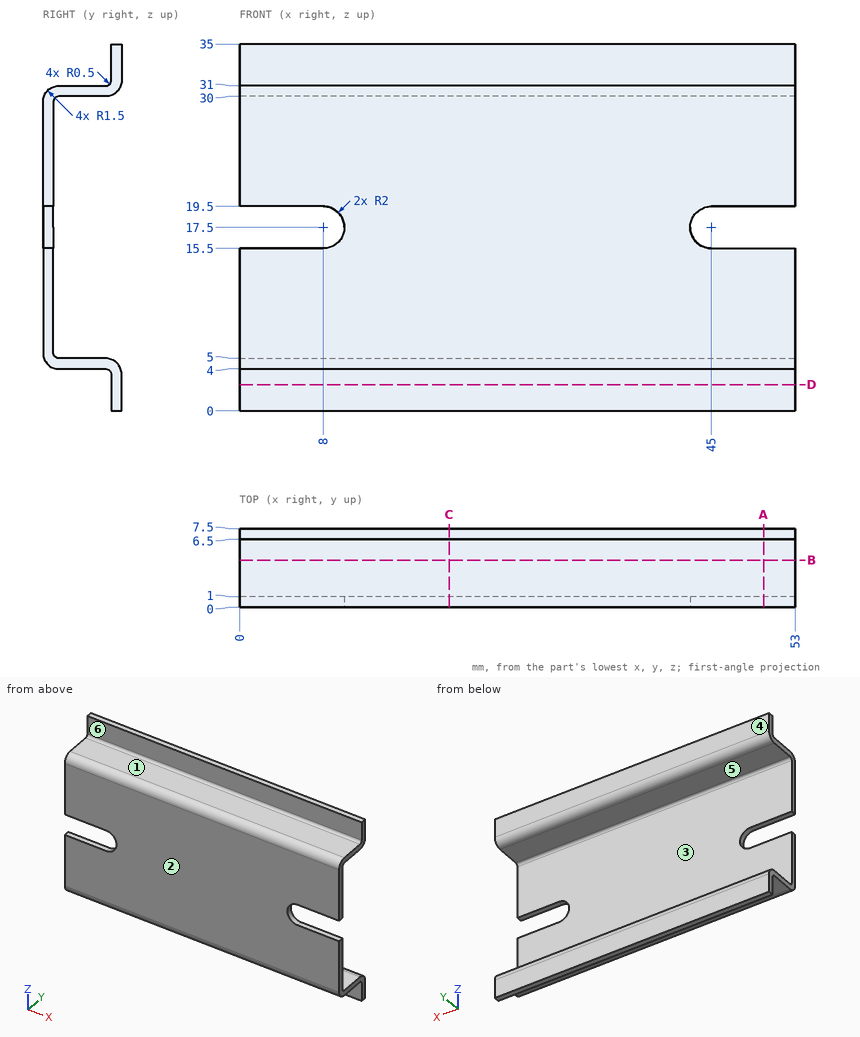
Study the drawing (mm; zero at the part's minimum x, y, z) and answer. A direction names the side the tool comes from. Coordinates: 2 decimals unless noted, no trailing zeros. Loops run counter-clockwise (first coordinate to the right, second up) from the corner with the lowest first, then second, coordinate; pieces in that order, holes last. Notation, with made-up numbers: M 23,20 L 34,20 A14 cw 34,41 Z; hole C 6.25,85 d8. An arc over 180 degrees is marked long. Answer in a Markdown table with one row per item. Add a question column.
1. Find section D-D, the plane z = 2.5. Write down the section's boundary in (x, y), then the cut area to 3 significant figures.
2. A tool of negligible diameter and unlimited length cuts with its end or side. For the marked faces 4, 5 and 6, from which of +Z, -Z, +X, -X, +Y, -Y can it reach the whole face along a straight path? Write none if from no direction.
3. Find section B-B, the plane y = 4.5. Write down the section's boundary in (x, z), then the cut area to 3 significant figures.
4. Consider L1, parallel to Z at x = 49, y = 4.25; L2, parallel to Y at x = 20, z = 26.5; L3, parallel to Z at x = 32, y = 1.25. Determine where each line is inside the solid, lowest interval first.
5. Find section C-C, the plane x = 20. Write down the section's boundary in (y, z).
6. Find section A-A, the plane x = 50. Write down the section's boundary in (y, z), then the cut area to 3 significant figures.
7. Flat-ended cylindrical pins translate along their axes: P1, Ø3.5, axis at x = 19.5, y = 3.5, coming from the +Z side; P2, Ø1, axis at x = 32.5, z = 2.5, coming from the -Y side; P3, Ø1.3, axis at x = 31, y = 3.5, coming from the -Z side. Find the tip coordinate at first contact, or state that the pin passes through.
8. The mould has two halves that part along Z. Classify the marked faces 1, 2 and 3: pulls with the +Z half, pulls with the -Z half, needs draft (parallel to the pull), parting line crosses it, or undercut.
Reported:
| question | item | result |
|---|---|---|
| 1 | outline | M 0,6.5 L 53,6.5 L 53,7.5 L 0,7.5 Z |
| 1 | area | 53.0 mm^2 |
| 2 | face 4 | +Z, -Z, +X, -X, +Y |
| 2 | face 5 | +X, -X, +Y |
| 2 | face 6 | +Z, +X, -X, -Y |
| 3 | outline | M 0,4 L 53,4 L 53,5 L 0,5 Z; M 0,30 L 53,30 L 53,31 L 0,31 Z |
| 3 | area | 106 mm^2 |
| 4 | L1 | z = 4 to 5, 30 to 31 |
| 4 | L2 | y = 0 to 1 |
| 4 | L3 | z = 4.02 to 5.07, 29.93 to 30.98 |
| 5 | outline | M 0,5.5 A1.5 ccw 1.5,4 L 6,4 A0.5 cw 6.5,3.5 L 6.5,0 L 7.5,0 L 7.5,3.5 A1.5 ccw 6,5 L 1.5,5 A0.5 cw 1,5.5 L 1,29.5 A0.5 cw 1.5,30 L 6,30 A1.5 ccw 7.5,31.5 L 7.5,35 L 6.5,35 L 6.5,31.5 A0.5 cw 6,31 L 1.5,31 A1.5 ccw 0,29.5 Z |
| 6 | outline | M 0,5.5 A1.5 ccw 1.5,4 L 6,4 A0.5 cw 6.5,3.5 L 6.5,0 L 7.5,0 L 7.5,3.5 A1.5 ccw 6,5 L 1.5,5 A0.5 cw 1,5.5 L 1,15.5 L 0,15.5 Z; M 0,19.5 L 1,19.5 L 1,29.5 A0.5 cw 1.5,30 L 6,30 A1.5 ccw 7.5,31.5 L 7.5,35 L 6.5,35 L 6.5,31.5 A0.5 cw 6,31 L 1.5,31 A1.5 ccw 0,29.5 Z |
| 6 | area | 42.3 mm^2 |
| 7 | P1 | stops at z = 31 |
| 7 | P2 | stops at y = 6.5 |
| 7 | P3 | stops at z = 4 |
| 8 | face 1 | pulls with the +Z half |
| 8 | face 2 | needs draft |
| 8 | face 3 | undercut |
